```python
from build123d import *

# Parameters (mm, degrees)
DODANIE_WYCI_GNI_CIE1_DEPTH       = 25
DODANIE_WYCI_GNI_CIE2_DEPTH       = 5
WYCI_GNI_CIE_CIENKA_START         = -70
WYCI_GNI_CIE_CIENKA_CIANKA1_DEPTH = 70
ZAOKR_GLENIE1_R                   = 10


with BuildPart() as part:
    # Szkic1 → Dodanie-wyci_gni_cie1 (new body)
    with BuildSketch(Plane.XY):
        with BuildLine():
            Line((0, 20), (0, 15))
            ThreePointArc((0, 15), (-15, 0), (0, -15))
            Line((0, -15), (0, -20))
            ThreePointArc((0, -20), (-20, 0), (0, 20))
        make_face()
    extrude(amount=DODANIE_WYCI_GNI_CIE1_DEPTH)

    # Szkic2 → Dodanie-wyci_gni_cie2 (add)
    with BuildSketch(Plane.XY):
        with BuildLine():
            Line((0, 20), (0, 72))
            Line((0, 72), (-40, 72))
            Line((-40, 72), (-40, 44.72135955))
            ThreePointArc((-40, 44.72135955), (-56.050341538, -21.409325386), (0, -60))
            Line((0, -60), (0, -20))
            ThreePointArc((0, -20), (-20, 0), (0, 20))
        make_face()
    extrude(amount=DODANIE_WYCI_GNI_CIE2_DEPTH)


with BuildPart() as body_2:
    # Lustro1: mirrored copy
    add(part.part.mirror(Plane.XY.offset(-35)))


with BuildPart() as part_1:
    add(part.part)

    add(body_2.part)  # Wyci_gni_cie-cienka _cianka1 merges body 2
    # Szkic3 → Wyci_gni_cie-cienka _cianka1 (add)
    with BuildSketch(Plane.XY.offset(WYCI_GNI_CIE_CIENKA_START)):
        with BuildLine():
            Line((-40, 72), (-40, 44.72135955))
            ThreePointArc((-40, 44.72135955), (-56.050341538, -21.409325386), (0, -60))
            Line((0, -60), (0, -55))
            ThreePointArc((0, -55), (-51.76124215, -18.594994247), (-35, 42.426406871))
            Line((-35, 42.426406871), (-35, 72))
            Line((-35, 72), (-40, 72))
        make_face()
    extrude(amount=WYCI_GNI_CIE_CIENKA_CIANKA1_DEPTH)

    # Zaokr_glenie1
    zaokr_glenie1_edges = [part_1.edges().sort_by_distance(p)[0] for p in [
        (-40, 58.360679775, 5),
        (-40, 58.360679775, -75),
    ]]
    fillet(zaokr_glenie1_edges, radius=ZAOKR_GLENIE1_R)


solid = part_1.part
```
The model under review builds one solid part; all positions refer to its coordinate system, in mm. A direction names the side the tool comes from. Give positions to 0.01 mm unless a question says otherwise; leave off trailing zeros. Write each loop counter-clockwise with the first axis right and the second up, starting at its lowest first coordinate (ties: lowest second). Pieces come first, ordered by that corner, then holes. Notation, with made-up numbers: (82, -22.75) -> (107, -22.75) arc R29 cw to (107, 9.25) -> close; hole circle Ø5 at (9, 48.5). An arc over 180 degrees is marked (long way). Answer in a Markdown table with one row per item.
1) For L1, parallel to Z at x = -4, y = -37.5; L2, parallel to Z at x = -47, y = -34; L3, parallel to Y at x = -44.5, z = -29, list the stretches that pass through material, from the lowest coordinate up. Write a range as [from, to].
Worked answers:
| item | result |
|---|---|
| L1 | [-75, -70], [0, 5] |
| L2 | [-75, 5] |
| L3 | [-40.25, -32.32], [32.32, 40.25] |
2) Mouldability with a two-part tool opening along Z and no side actions: class faces 4 (the flat face through (-22, 9, 0)), 5 (the flat face through (-15.1, -1.4, 25)), 6 (the cylindrical face through (-15, 0, 12)) as +Z half, -Z half, draft (parallel to the pull), parting line (faces both ways), or undercut.
Worked answers:
| item | result |
|---|---|
| face 4 | undercut |
| face 5 | +Z half |
| face 6 | draft |
3) Tool access review of faces 1 (the flat face through (-40, 59, -35)), 2 (the flat face through (-22, 9, -70)), 3 (the cylindrical face through (-37.15, 58.17, -71.99)): name each direction out of +Z, -Z, +X, -X, +Y, -Y from which nothing blocks a thin tool from reaching the whole face with its end or side.
Worked answers:
| item | result |
|---|---|
| face 1 | +Z, -Z, -X, +Y |
| face 2 | +X |
| face 3 | -Z, -X, +Y |
4) Add section B-B on x = -7.5. State the section outline as (y, z) points.
Worked answers:
| item | result |
|---|---|
| outline | (-59.53, -75) -> (-18.54, -75) -> (-18.54, -95) -> (-12.99, -95) -> (-12.99, -70) -> (-54.49, -70) -> (-54.49, 0) -> (-12.99, 0) -> (-12.99, 25) -> (-18.54, 25) -> (-18.54, 5) -> (-59.53, 5) -> close; (12.99, -95) -> (18.54, -95) -> (18.54, -75) -> (72, -75) -> (72, -70) -> (12.99, -70) -> close; (12.99, 0) -> (72, 0) -> (72, 5) -> (18.54, 5) -> (18.54, 25) -> (12.99, 25) -> close |
5) Clearance check with flat-ended pins moving along their axes: P1, Ø1.5, axis at y = 57, z = -73.5, coming from the -X side; P2, Ø8, axis at y = 53, z = -36.5, coming from the -X side; P3, Ø12, axis at x = -44, y = -16.5, coming from the -Z side. State where each tip first meets the part, or that it passes through.
Worked answers:
| item | result |
|---|---|
| P1 | x = -36.32 |
| P2 | x = -40 |
| P3 | z = -75 |
6) Add section D-D on y = 39. State the section outline as (x, z) points.
Worked answers:
| item | result |
|---|---|
| outline | (-45.6, -75) -> (0, -75) -> (0, -70) -> (-38.78, -70) -> (-38.78, 0) -> (0, 0) -> (0, 5) -> (-45.6, 5) -> close |
7) Add section C-C on z = -29.5. State the section outline as (x, y) points.
Worked answers:
| item | result |
|---|---|
| outline | (-40, 44.72) arc R60 ccw to (0, -60) -> (0, -55) arc R55 cw to (-35, 42.43) -> (-35, 72) -> (-40, 72) -> close |
8) Add section A-A on y = 0. State the section outline as (x, z) points, plus the area to 3 significant figures.
Worked answers:
| item | result |
|---|---|
| outline | (-60, -75) -> (-20, -75) -> (-20, -95) -> (-15, -95) -> (-15, -70) -> (-55, -70) -> (-55, 0) -> (-15, 0) -> (-15, 25) -> (-20, 25) -> (-20, 5) -> (-60, 5) -> close |
| area | 1,000 mm² |
